Study the drawing (mm; zero at the part's minimum x, y, z) and answer. A direction names the side the tool comes from. Give positions to 0.01 mm unless a question says otherwise; leave off trailing zeros. Order: outer loops, then holes, each group sorted by start corner. A loop starts at its lowest first (then second) coordinate and runs counter-clockwise, first axis right, second up. Notation, with made-up numbers: (-13.5, -26) - (10.5, -26) arc R31 cw to (10.5, 11) - close; hole circle Ø11 at (86.5, 42.25). An arc over 180 degrees is marked (long way). Use CSV: the item, a comma, the result in double quotes.
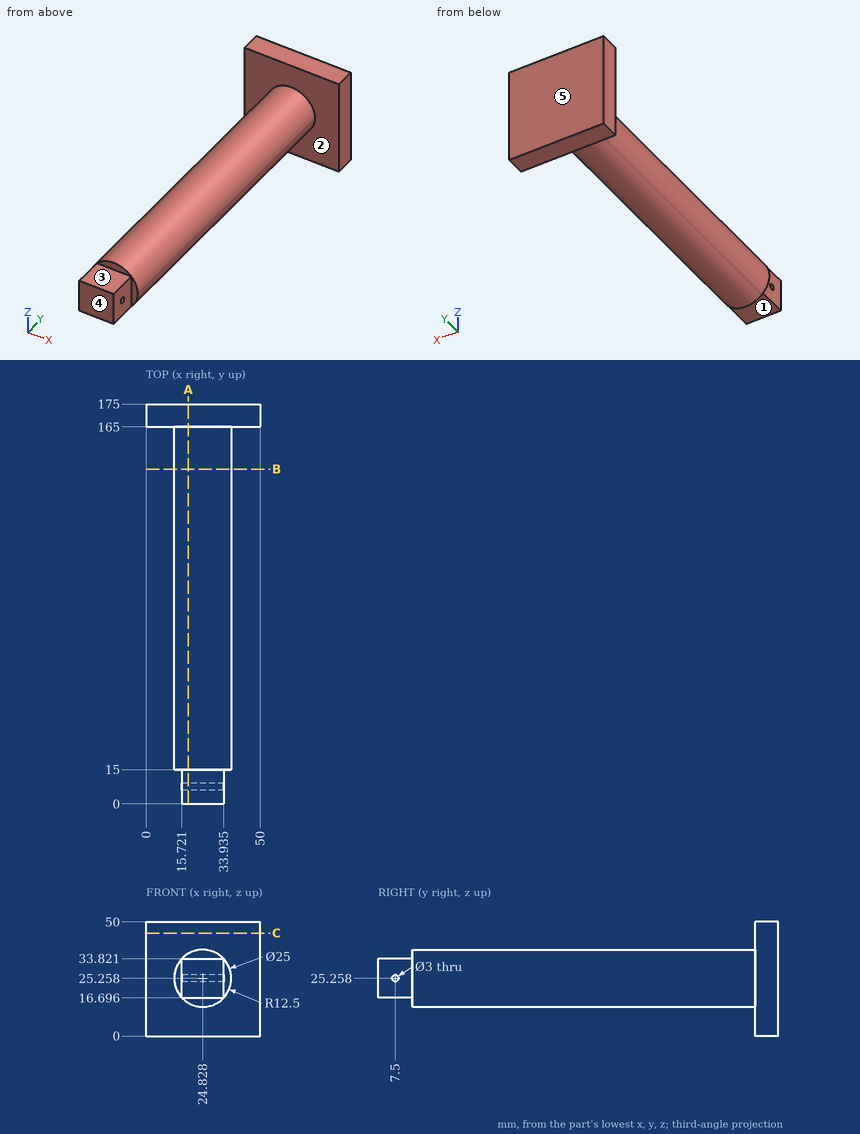
Item 1: Find the intervals of material crossed by line 1 along Z through (x, y) = (26.75, 7.5); line 2 along Y through (x, z) = (15, 17); line 3 along Z through (x, y) = (22, 7) (1 decimal), in increasing order.
Taken from the geometry:
line 1,"16.7 to 23.76, 26.76 to 33.82"
line 2,"165 to 175"
line 3,"16.7 to 23.8, 26.7 to 33.8"
Item 2: The part is cut by section A-A (x = 18.5). Give the vertices of the cut face in (y, z).
Taken from the geometry:
outline,"(0, 16.7) - (15, 16.7) - (15, 14.48) - (165, 14.48) - (165, 0) - (175, 0) - (175, 50) - (165, 50) - (165, 36.04) - (15, 36.04) - (15, 33.82) - (0, 33.82) - close; hole circle Ø3 at (7.5, 25.26)"
Item 3: The part is cut by section B-B (y = 146.5). Give the vertices of the cut face in (x, z).
Taken from the geometry:
outline,"circle Ø25 at (24.83, 25.26)"
Item 4: Which of the six approach directions +Z, -Z, +X, -X, +Y, -Y give full straight-line access (tool end or side, diameter ignored) to the marked faces 1, 2, 3, 4 and 5?
Taken from the geometry:
face 1,"-Z, +X, -X, -Y"
face 2,"-Y"
face 3,"+Z, +X, -X, -Y"
face 4,"+Z, -Z, +X, -X, -Y"
face 5,"+Z, -Z, +X, -X, +Y"
Item 5: Each of these flat-tipped pins is pushed along its axis until it touches: pin 1 (12 mm diameter, centred on x = 26.5, y = 9.5, fed in from -Z); pin 2 (10 mm diameter, centred on x = 35.5, y = 142.5, fed in from +Z); pin 3 (3.5 mm diameter, centred on y = 7.5, z = 25.26, fed in from +X) (1 decimal); pin 4 (4 mm diameter, centred on x = 39.5, y = 98, fed in from -Z). Where does it stop, or does it pass through?
Taken from the geometry:
pin 1,"z = 12.76"
pin 2,"z = 36.4"
pin 3,"x = 33.9"
pin 4,"through"
Item 6: The part is cut by section C-C (z = 45). Give the vertices of the cut face in (x, y), and give its area (3 significant figures).
Taken from the geometry:
outline,"(0, 165) - (50, 165) - (50, 175) - (0, 175) - close"
area,"500 mm^2"
